from build123d import *

# Parameters (mm, degrees)
F1_DEPTH = 14
F3_W     = 25
F3_H     = 2
F4_DEPTH = 6
F5_W     = 25
F5_H     = 2
F6_DEPTH = 6
F8_D     = 3.5
F10_D    = 3.5
F11_D    = 12.75


with BuildPart() as f1:
    # F0 (on Top) → F1 (new body)
    with BuildSketch(Plane.XY):
        Polygon((12.5, 0), (0, 0), (-12.5, 0), (-12.5, -2), (12.5, -2), align=None)
        Polygon((-12.5, 0), (0, 0), (12.5, 0), (7, 7), (0, 7), (-7, 7), align=None)
    extrude(amount=F1_DEPTH)

    # F3 (on face) → F4 (join)
    with BuildSketch(Plane(origin=(0, 0, 0), x_dir=(1, 0, 0), z_dir=(0, 0, -1))):
        with Locations((0, 1)):
            Rectangle(F3_W, F3_H)
    extrude(amount=F4_DEPTH)

    # F5 (on face) → F6 (join)
    with BuildSketch(Plane.XY.offset(14)):
        with Locations((0, -1)):
            Rectangle(F5_W, F5_H)
    extrude(amount=F6_DEPTH)

    # F8 (through all)
    with Locations(Plane(origin=(0, 0, 0), x_dir=(-1, 0, 0), z_dir=(0, 1, 0))):
        with Locations((0, -3.387567)):
            Hole(F8_D / 2)

    # F10 (through all)
    with Locations(Plane(origin=(0, 0, 0), x_dir=(-1, 0, 0), z_dir=(0, 1, 0))):
        with Locations((0, 17.537134)):
            Hole(F10_D / 2)

    # F11 (through all)
    with Locations(Plane(origin=(0, 7, 0), x_dir=(-1, 0, 0), z_dir=(0, 1, 0))):
        with Locations((0, 7)):
            Hole(F11_D / 2)


solid = f1.part
The listing builds one solid part. Answer for the finished solid, in the listing's coordinates (mm). A direction names the side the tool comes from. Coordinates: 2 decimals unless noted, no trailing zeros. Loops run counter-clockwise (first coordinate to the right, second up) from the corner with the lowest first, then second, coordinate; pieces in that order, holes last. Notation, with made-up numbers: M 75,74.5 L 109,74.5 A8 ccw 109,89.5 Z; hole C 83.5,-24.5 d2. An arc over 180 degrees is marked long. Answer in a Markdown table with one row per item.
1) Find the intervals of material crossed by probe 1 along Z at (x, y) = (0, -1.3) (3 decimals); probe 2 along Y at (x, z) = (9.5, 15.75); probe 3 along X at (y, z) = (4.5, 12.5), in increasing order.
Answers below:
| item | result |
|---|---|
| probe 1 | -6 to -5.138, -1.638 to 0.625, 13.375 to 15.787, 19.287 to 20 |
| probe 2 | -2 to 0 |
| probe 3 | -8.96 to -3.22, 3.22 to 8.96 |
2) Find section B-B (z = 12.75). Determine the outline of the cut face in (x, y).
Answers below:
| item | result |
|---|---|
| outline | M -12.5,-2 L -2.75,-2 L -2.75,7 L -7,7 L -12.5,0 Z; M 2.75,-2 L 12.5,-2 L 12.5,0 L 7,7 L 2.75,7 Z |
3) Find section D-D (y = 6.5). Determine the outline of the cut face in (x, z) (3 decimals), then the cut area to 3 significant figures.
Answers below:
| item | result |
|---|---|
| outline | M -7.393,0 L 7.393,0 L 7.393,14 L -7.393,14 Z; hole C 0,7 d12.75 |
| area | 79.3 mm^2 |
4) Find section A-A (x = 0). Determine the outline of the cut face in (y, z) (3 decimals).
Answers below:
| item | result |
|---|---|
| outline | M -2,-6 L 0,-6 L 0,-5.138 L -2,-5.138 Z; M -2,-1.638 L 0,-1.638 L 0,0 L 7,0 L 7,0.625 L -2,0.625 Z; M -2,13.375 L 7,13.375 L 7,14 L 0,14 L 0,15.787 L -2,15.787 Z; M -2,19.287 L 0,19.287 L 0,20 L -2,20 Z |
5) Determine the mould class of faces 4 (the flat face through (0, -1, 20)), 5 (the flat face through (12.5, -1, 7)), 6 (the cylindrical face through (1.67, -1.01, -2.86)) for opening direction Z: released by +Z, released by -Z, zero draft, split by the parting line, or undercut.
Answers below:
| item | result |
|---|---|
| face 4 | released by +Z |
| face 5 | zero draft |
| face 6 | undercut |
6) Given pin 1 (3 mm diameter, centred on x = 0, z = -4, fed in from +Y); pin 2 (2 mm diameter, centred on x = 5.5, y = 2, fed in from -Z); pin 3 (2 mm diameter, centred on x = 2.5, y = 2.5, fed in from +Z); pin 4 (11.5 mm diameter, centred on x = 0, z = 7, fed in from +Y), each flat-ended and moving along its own axis, determine where each tip first touches the part or whether it passes through.
Answers below:
| item | result |
|---|---|
| pin 1 | y = 0 |
| pin 2 | z = 0 |
| pin 3 | z = 14 |
| pin 4 | through |
7) Which of the six approach directions +Z, -Z, +X, -X, +Y, -Y give full straight-line access (tool end or side, diameter ignored) to faces 1 (the flat face through (0, 0, -1)), 2 (the flat face through (-12.5, -1, 7)), 3 (the flat face through (-0.2, 0, 15.6))?
Answers below:
| item | result |
|---|---|
| face 1 | -Z, +X, -X, +Y |
| face 2 | +Z, -Z, -X, +Y, -Y |
| face 3 | +Z, +X, -X, +Y |
8) Find section C-C (x = -5.5). Determine the outline of the cut face in (y, z), then the cut area to 3 significant figures.
Answers below:
| item | result |
|---|---|
| outline | M -2,-6 L 0,-6 L 0,0 L 7,0 L 7,3.78 L -2,3.78 Z; M -2,10.22 L 7,10.22 L 7,14 L 0,14 L 0,20 L -2,20 Z |
| area | 92.0 mm^2 |
